Source: CAD feature listing. Evaluate the final solid. Frame: model axes, mm. A direction names the side the tool comes from. Give positions to 0.01 mm unless a question says otherwise; leave off trailing zeros. Loops run counter-clockwise (first coordinate to the right, second up) from the corner with the lowest first, then second, coordinate; pieces in that order, holes last. Notation, with made-up numbers: (-12.75, 41) -> (-4.75, 41) arc R23 cw to (-4.75, 76) -> close; hole circle Ø4 at (70.25, 64.25). An arc over 180 degrees is marked (long way). Put each result on its own line as item: value.
```python
from build123d import *

# Parameters (mm, degrees)
BOSS_EXTRUDE1_DEPTH = 0.8
SKETCH2_R           = 1
BOSS_EXTRUDE2_DEPTH = 2
SKETCH3_R           = 2
BOSS_EXTRUDE3_DEPTH = 3.26
SKETCH6_R           = 2
BOSS_EXTRUDE4_DEPTH = 3.34


with BuildPart() as part:
    # Sketch1 → Boss-Extrude1 (new body)
    with BuildSketch(Plane.XY):
        with BuildLine():
            Line((-2.002843202, 5.298630925), (-4.336792166, -3.276937888))
            ThreePointArc((-4.336792166, -3.276937888), (-4.27139076, -4.52603882), (-3.476760681, -5.492006479))
            ThreePointArc((-3.476760681, -5.492006479), (0, -6.5), (3.476760681, -5.492006479))
            ThreePointArc((3.476760681, -5.492006479), (4.27139076, -4.52603882), (4.336792166, -3.276937888))
            Line((4.336792166, -3.276937888), (2.002843202, 5.298630925))
            ThreePointArc((2.002843202, 5.298630925), (1.489063424, 6.102778606), (0.608877551, 6.471419329))
            ThreePointArc((0.608877551, 6.471419329), (0, 6.5), (-0.608877551, 6.471419329))
            ThreePointArc((-0.608877551, 6.471419329), (-1.489063424, 6.102778606), (-2.002843202, 5.298630925))
        make_face()
    extrude(amount=BOSS_EXTRUDE1_DEPTH)

    # Sketch2 → Boss-Extrude2 (add)
    with BuildSketch(Plane.XY.offset(0.8)):
        with Locations((0, 5.26)):
            Circle(SKETCH2_R)
    extrude(amount=BOSS_EXTRUDE2_DEPTH)

    # Sketch3 → Boss-Extrude3 (add)
    with BuildSketch(Plane(origin=(0, 0, 0), x_dir=(-1, 0, 0), z_dir=(0, 0, -1))):
        Circle(SKETCH3_R)
    extrude(amount=BOSS_EXTRUDE3_DEPTH)

    # Mirror1: part across plane


with BuildPart() as part_1:
    add(part.part)
    add(part.part.mirror(Plane(origin=(0, 5.26, 2.8), x_dir=(1, 0, 0), z_dir=(0, 0, 1))))

    # Sketch6 → Boss-Extrude4 (add)
    with BuildSketch(Plane.XY.offset(8.86)):
        Circle(SKETCH6_R)
    extrude(amount=BOSS_EXTRUDE4_DEPTH)


solid = part_1.part
```
(1) Section A-A on x = 2.25. Return loops of the section in (y, z).
Calculated:
outline: (-6.1, 0) -> (4.39, 0) -> (4.39, 0.8) -> (-6.1, 0.8) -> close; (-6.1, 4.8) -> (4.39, 4.8) -> (4.39, 5.6) -> (-6.1, 5.6) -> close
(2) First-contact query: P1, Ø5, axis at x = 0, z = 4, coming from the +Y side; P2, Ø1, axis at x = -3, y = -2.5, coming from the +Z side; P3, Ø4, axis at y = 0, z = 6, coming from the -X side; P4, Ø1.5, axis at x = 2.5, z = 0, coming from the +Y side. Flat tips, straight axial feed; report the tip coordinate or a pass-through.
Calculated:
P1: stops at y = 6.5
P2: stops at z = 5.6
P3: stops at x = -3.98
P4: stops at y = 5.82
(3) Line query: probe 1 along Z at (x, y) = (-2, 2); probe 2 along Z at (x, y) = (0, 1); probe 3 along X at (y, z) = (6, 1.5). Output: solid intervals per line, ascending. Write a range as from..to.
Calculated:
probe 1: z = 0..0.8, 4.8..5.6
probe 2: z = -3.26..0.8, 4.8..12.2
probe 3: x = -0.67..0.67
(4) Section D-D on y = 4. Return loops of the section in (x, z).
Calculated:
outline: (-2.36, 0) -> (2.36, 0) -> (2.36, 0.8) -> (-2.36, 0.8) -> close; (-2.36, 4.8) -> (2.36, 4.8) -> (2.36, 5.6) -> (-2.36, 5.6) -> close
(5) Draft query along Z for faces 3 (the flat face through (0, -1, 4.8)), 4 (the flat face through (0, -3, 0)), 5 (the flat face through (3.186, 0.951, 0.394)). Return one class per face: released by +Z, released by -Z, zero draft, split by the parting line, or undercut.
Calculated:
face 3: undercut
face 4: released by -Z
face 5: zero draft
(6) Section C-C on x = 0. Return loops of the section in (y, z).
Calculated:
outline: (-6.5, 0) -> (-2, 0) -> (-2, -3.26) -> (2, -3.26) -> (2, 0) -> (6.5, 0) -> (6.5, 0.8) -> (6.26, 0.8) -> (6.26, 4.8) -> (6.5, 4.8) -> (6.5, 5.6) -> (2, 5.6) -> (2, 12.2) -> (-2, 12.2) -> (-2, 5.6) -> (-6.5, 5.6) -> (-6.5, 4.8) -> (4.26, 4.8) -> (4.26, 0.8) -> (-6.5, 0.8) -> close
(7) Section B-B on y = 0. Return loops of the section in (x, z).
Calculated:
outline: (-3.44, 0) -> (-2, 0) -> (-2, -3.26) -> (2, -3.26) -> (2, 0) -> (3.44, 0) -> (3.44, 0.8) -> (-3.44, 0.8) -> close; (-3.44, 4.8) -> (3.44, 4.8) -> (3.44, 5.6) -> (2, 5.6) -> (2, 12.2) -> (-2, 12.2) -> (-2, 5.6) -> (-3.44, 5.6) -> close
(8) Reachability of faces 1 (the cylindrical face through (1.499, 6.094, 0.394)), 2 (the cylindrical face through (0, -2, -2)) from +Z, -Z, +X, -X, +Y, -Y: full face, straight path, thin tool, end or side. Return the list, or none.
Calculated:
face 1: +Z, -Z, +X, +Y
face 2: -Z
